Verification items for the finished model (mm, model axes). Round coordinates to 2 decimals unless told otherwise and drop trailing zeros. Order: outer loops, then holes, each group sorted by start corner. A loop starts at its lowest first (then second) coordinate and runs counter-clockwise, first axis right, second up. Notation, with made-up numbers: (16, -24) -> (20, -24) arc R21 cw to (20, -15) -> close; hole circle Ø4 at (11.5, -17.75). An arc over 180 degrees is marked (long way). Put each result on its own line as item: value.
from build123d import *

# Parameters (mm, degrees)
F0_R     = 6.35
F1_DEPTH = 4.7625


with BuildPart() as f1:
    # F0 (on Right) → F1 (new body, symmetric)
    with BuildSketch(Plane.YZ):
        with BuildLine():
            Line((-217.446472, -20.817392), (163.553528, -20.817392))
            ThreePointArc((163.553528, -20.817392), (182.603528, -1.767392), (163.553528, 17.282608))
            Line((163.553528, 17.282608), (-217.446472, 17.282608))
            ThreePointArc((-217.446472, 17.282608), (-236.496472, -1.767392), (-217.446472, -20.817392))
        make_face()
        with Locations((-217.446472, -1.767392)):
            Circle(F0_R, mode=Mode.SUBTRACT)
        with Locations((163.553528, -1.767392)):
            Circle(F0_R, mode=Mode.SUBTRACT)
    extrude(amount=F1_DEPTH, both=True)


solid = f1.part
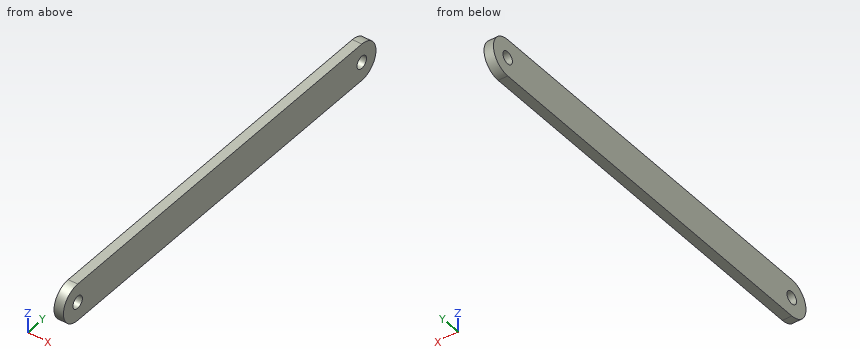
Item 1: Section check B-B on z = 13.5. Record the boundary of the cut face in (x, y), then the cut area to 3 significant figures.
Check sheet entries:
outline: (-4.76, -228.84) -> (4.76, -228.84) -> (4.76, 174.95) -> (-4.76, 174.95) -> close
area: 3,850 mm^2
Item 2: Section check A-A on x = 2.25. Record the boundary of the cut face in (y, z), then the cut area to 3 significant figures.
Check sheet entries:
outline: (-217.45, -20.82) -> (163.55, -20.82) arc R19.05 ccw to (163.55, 17.28) -> (-217.45, 17.28) arc R19.05 ccw to start; hole circle Ø12.7 at (-217.45, -1.77); hole circle Ø12.7 at (163.55, -1.77)
area: 15,400 mm^2
Item 3: Material ranges on L1, parallel to Y at x = -3.5, z = -2; L2, parallel to Y at x = 2.75, z = 3.5; L3, parallel to Y at x = -2.5, z = 6, recorded low to high. Write a range as [from, to].
Check sheet entries:
L1: y = [-236.5, -223.79], [-211.1, 157.21], [169.9, 182.6]
L2: y = [-235.75, -220.99], [-213.9, 160.01], [167.1, 181.86]
L3: y = [-234.84, 180.95]
Item 4: Gauge pin test, flat ends, axial feed: pin 1 Ø1 at (x, z) = (3, 2) entering from +Y; pin 2 Ø2 at (x, z) = (-3, 0.5) entering from +Y; pin 3 Ø5 at (x, z) = (3.5, 12) entering from -Y; pin 4 Ø7.5 at (y, z) = (-217.45, -1.77) entering from +X. Record the tip position at first contact, or that the pin passes through.
Check sheet entries:
pin 1: stops at y = 182.32
pin 2: stops at y = 182.56
pin 3: stops at y = -232.81
pin 4: passes through
Item 5: Section check C-C on z = -13. Record the boundary of the cut face in (x, y), then the cut area to 3 significant figures.
Check sheet entries:
outline: (-4.76, -232.83) -> (4.76, -232.83) -> (4.76, 178.94) -> (-4.76, 178.94) -> close
area: 3,920 mm^2
